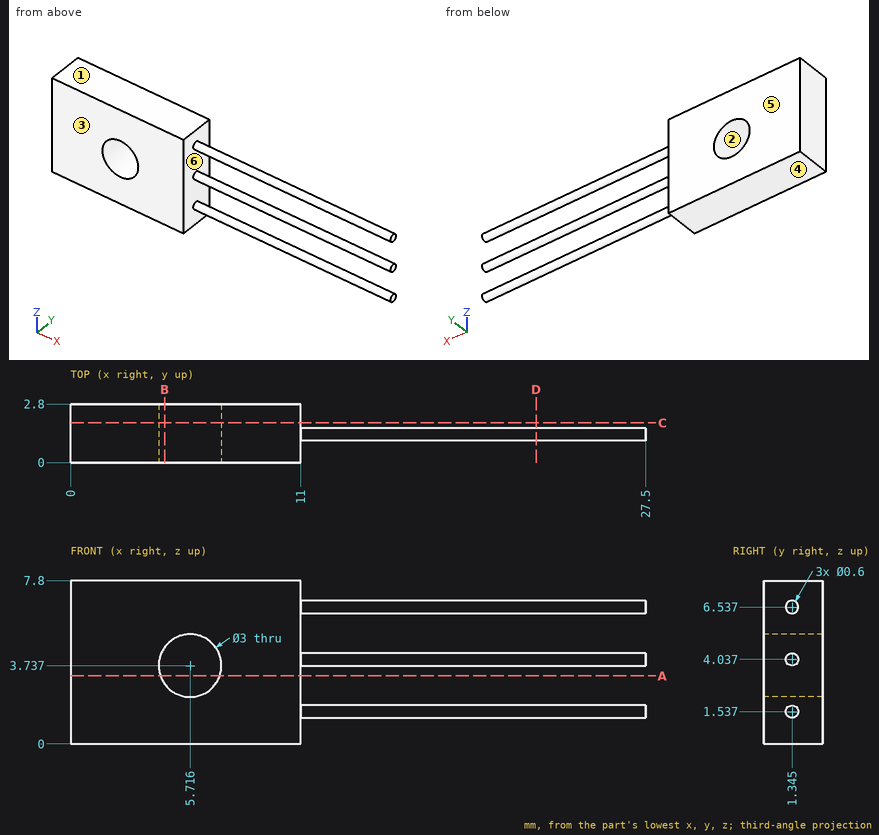
The figure shows three views and two pictorial views of one solid part (mm, origin at its lowest corner). Answer the questions. A direction names the side the tool comes from. Give positions to 0.01 mm unless a question says otherwise; leave off trailing zeros. Loops run counter-clockwise (first coordinate to the right, second up) from the corner with the lowest first, then second, coordinate; pieces in that order, holes last. Notation, with made-up numbers: M -24.75,61.5 L -7.75,61.5 A21 cw -7.75,96.5 Z; hole C 55.5,-3 d6. An arc over 180 degrees is marked long. Write each question's results on one line, items separated by ' | '.
1. Given pin 1 (2 mm diameter, centred on x = 23, z = 5, fed in from +Y) (1 decimal); pin 2 (0.8 mm diameter, centred on y = 1.5, z = 3, fed in from +X), each flat-ended and moving along its own axis, determine where each tip first touches the part or whether it passes through.
Values:
pin 1: stops at y = 1.6 | pin 2: stops at x = 11
2. Straight lines are drawn through the part: line 1 (X direction, y = 1, z = 6); line 2 (Z direction, x = 11.75, y = 1.45) (1 decimal); line 3 (Y direction, x = 16, z = 1.5). For each, find the intervals that lie inside material, in ascending order. Write a range as [from, to].
Values:
line 1: x = [0, 11] | line 2: z = [1.3, 1.8], [3.8, 4.3], [6.3, 6.8] | line 3: y = [1.05, 1.64]
3. Section C-C on y = 1.9 is taken. Give the vertices of the cut face in (x, z) (1 decimal).
Values:
outline: M 0,0 L 11,0 L 11,7.8 L 0,7.8 Z; hole C 5.7,3.7 d3
4. Section A-A on z = 3.25 is taken. Give the vertices of the cut face in (x, y) (1 decimal).
Values:
outline: M 0,0 L 4.3,0 L 4.3,2.8 L 0,2.8 Z; M 7.1,0 L 11,0 L 11,2.8 L 7.1,2.8 Z
5. Section B-B on x = 4.5 is taken. Give the vertices of the cut face in (y, z).
Values:
outline: M 0,0 L 2.8,0 L 2.8,2.86 L 0,2.86 Z; M 0,4.62 L 2.8,4.62 L 2.8,7.8 L 0,7.8 Z
6. The mould has two halves that part along Z. Classify the marked faces 1, 2, 3 and 4: pulls with the +Z half, pulls with the -Z half, needs draft (parallel to the pull), parting line crosses it, or undercut.
Values:
face 1: pulls with the +Z half | face 2: undercut | face 3: needs draft | face 4: pulls with the -Z half
7. A tool of negligible diameter and unlimited length cuts with its end or side. For the marked faces 5 and 6, from which of +Z, -Z, +X, -X, +Y, -Y can it reach the whole face along a straight path? Write none if from no direction.
Values:
face 5: +Z, -Z, +X, -X, +Y | face 6: +X
8. Section D-D on x = 22.25 is taken. Give the vertices of the cut face in (y, z) (1 decimal).
Values:
outline: C 1.3,1.5 d0.6; C 1.3,4 d0.6; C 1.3,6.5 d0.6
